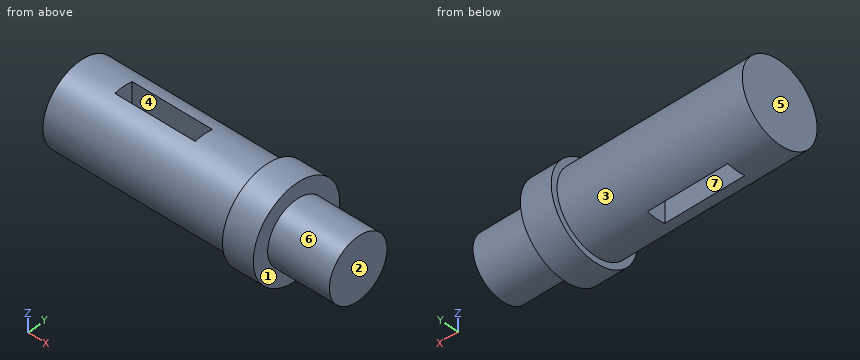
Solid Edge part; units mm, degrees
sketch "Sketch1" plane through (0, 0, 0) normal (1, 0, 0) x (0, 1, 0)
  circle A0 centre (0, 0) radius 10
extrude "Protrusion1" add sketch "Sketch1" against normal blind 20
sketch "Sketch2" plane through (-20, 0, 0) normal (-1, 0, 0) x (0, 1, 0)
  circle A0 centre (0, 0) radius 15
extrude "ExtrudedProtrusion_2" add sketch "Sketch2" along normal blind 10
sketch "Sketch3" plane through (-30, 0, 0) normal (-1, 0, 0) x (0, 1, 0)
  circle A0 centre (0, 0) radius 13
extrude "ExtrudedProtrusion_3" add sketch "Sketch3" along normal blind 60
sketch "Sketch4" plane through (0, 0, 0) normal (0, 0, 1) x (1, 0, 0)
  line L0 (-76, 3) -> (-50, 3)
  line L1 (-50, 3) -> (-50, -3)
  line L2 (-50, -3) -> (-76, -3)
  line L3 (-76, -3) -> (-76, 3)
  dimension "D1" = 76
  dimension "D2" = 76
extrude "ExtrudedCutout_1" cut sketch "Sketch4" along normal mid plane 78.6359
properties part number "2"
Geometry check sheet. Reference: the model listing, model coordinates, mm. Face numbers are marked on the shaded views. A direction names the side the tool comes from. Coordinates: 2 decimals unless noted, no trailing zeros. Write each loop counter-clockwise with the first axis right and the second up, starting at its lowest first coordinate (ties: lowest second). Pieces come first, ordered by that corner, then holes. Notation, with made-up numbers: (-29, -34) -> (-13, -34) arc R15 ccw to (-13, -26) -> close; hole circle Ø2 at (30.5, 71.5). An arc over 180 degrees is marked (long way). One line per question, with ' | ' between items.
1. Cross-section at D-D on y = -6. Record the cut outline in (x, z), and give its area (3 significant figures).
Answers:
outline: (-90, -11.53) -> (-30, -11.53) -> (-30, -13.75) -> (-20, -13.75) -> (-20, -8) -> (0, -8) -> (0, 8) -> (-20, 8) -> (-20, 13.75) -> (-30, 13.75) -> (-30, 11.53) -> (-90, 11.53) -> close | area: 1,980 mm²
2. Thickness scan on probe 1 along X at (y, z) = (1.75, 3.5); probe 2 along X at (y, z) = (-7.75, -8.5); probe 3 along Z at (x, y) = (-10.5, -0.25). Record the ranges inside material, lowest first. Write a range as from..to.
Answers:
probe 1: x = -90..-76, -50..0 | probe 2: x = -90..-20 | probe 3: z = -10..10
3. Cross-section at A-A on y = 0. Record the cut outline in (x, z), and give its area (3 significant figures).
Answers:
outline: (-90, -13) -> (-76, -13) -> (-76, 13) -> (-90, 13) -> close; (-50, -13) -> (-30, -13) -> (-30, -15) -> (-20, -15) -> (-20, -10) -> (0, -10) -> (0, 10) -> (-20, 10) -> (-20, 15) -> (-30, 15) -> (-30, 13) -> (-50, 13) -> close | area: 1,580 mm²
4. Set-up check for the marked faces 1, 2, 3 and 4: record each of +Z, -Z, +X, -X, +Y, -Y from which the full face is reachable in a straight line by a thin tool's end or side.
Answers:
face 1: +X | face 2: +Z, -Z, +X, +Y, -Y | face 3: -X | face 4: +Z, -Z
5. Depth check by flat-ended pin: pin 1 Ø3 at (x, y) = (-74.5, 11) entering from -Z; pin 2 Ø6 at (x, z) = (-21.5, -8.5) entering from -Y; pin 3 Ø3 at (x, y) = (-56, -7.5) entering from -Z; pin 4 Ø2 at (x, y) = (-52, -0.5) entering from -Z. Enter the tip coordinate at first touch or a pass-through.
Answers:
pin 1: stops at z = -8.87 | pin 2: stops at y = -13.96 | pin 3: stops at z = -11.53 | pin 4: passes through
6. Cross-section at C-C on x = -28. Record the cut outline in (y, z).
Answers:
outline: circle Ø30 at (0, 0)
7. Draft check along Y on the marked faces 5, 6 and 7. Enter one of: +Y half, -Y half, draft (parallel to the pull), parting line (faces both ways), or undercut.
Answers:
face 5: draft | face 6: parting line | face 7: undercut
8. Cross-section at B-B on z = 0. Record the cut outline in (x, y).
Answers:
outline: (-90, -13) -> (-30, -13) -> (-30, -15) -> (-20, -15) -> (-20, -10) -> (0, -10) -> (0, 10) -> (-20, 10) -> (-20, 15) -> (-30, 15) -> (-30, 13) -> (-90, 13) -> close; hole (-76, -3) -> (-50, -3) -> (-50, 3) -> (-76, 3) -> close
